Here's how the part is built. I have some questions about the finished solid (model axes, mm). A direction names the side the tool comes from. Round coordinates to 2 decimals unless told otherwise and drop trailing zeros. Loops run counter-clockwise (first coordinate to the right, second up) from the corner with the lowest first, then second, coordinate; pieces in that order, holes last. Notation, with made-up numbers: (-8.75, -9) - (0.25, -9) arc R16 ccw to (0.25, -3) - close; hole circle Ø5 at (89, 71.25). An arc over 180 degrees is marked (long way). Answer as a JSON object with one key per item and string values. Group by question number.
1) If we mould it in two halves opening along X, with no side actions, what happens to faces 4 (the face through (1.902, 0.986, -5.739)), 5 (the face through (0, 1, 16)), 6 (the face through (-4.766, 0.986, -1.475)), 7 (the face through (0, 8, 9))? For each: pulls with the +X half, pulls with the -X half, needs draft (parallel to the pull), parting line crosses it, or undercut.
2) I want a section at A-A, the plane z = 0. Please give me the cut outline in (x, y), then the cut area to 3 significant figures.
3) I want a section at C-C, the plane y = 1. Please give me the cut outline in (x, z), then the cut area to 3 significant figures.
4) If I drill on line 1 along X through (y, z) = (1.25, 0); line 2 along Z through (x, y) = (0, 0.5); line 3 along Y through (x, z) = (2, 14), over which ranges is the centre line in solid material (lowest first)? Write a range as [from, to].
5) Will these pins go through, and if not, where does the flat tip stop? P1, Ø4, axis at x = 0.5, z = 5.5, coming from the -Y side; P2, Ø2, axis at x = -5, y = 2, coming from the +Z side; P3, Ø1.6, axis at y = 1, z = 11.5, coming from the -X side; P4, Ø4, axis at x = -1, y = 7, coming from the -Z side.
6) Which directions (+Z, -Z, +X, -X, +Y, -Y) give clear straight access to the entire face, cutting with the end or side of a thin tool? Please do faces 1 (the face through (0.11, 7.415, 11.748)), 2 (the face through (-3, 1, 10)), 3 (the face through (3, 1, 10)).
7) I want a section at B-B, the plane x = -5. Please give me the cut outline in (y, z), then the cut area to 3 significant figures.
8) I want a section at D-D, the plane z = 9.25. Please give me the cut outline in (x, y), then the cut area to 3 significant figures.
from build123d import *

# Parameters (mm, degrees)
SKETCH_1_R      = 2
EXTRUDE_1_DEPTH = 2
SKETCH_2_R      = 2.5
EXTRUDE_2_DEPTH = 8


with BuildPart() as part:
    # 草图1 → 凸台-拉伸1 (new body)
    with BuildSketch(Plane(origin=(0, 0, 0), x_dir=(1, 0, 0), z_dir=(0, 1, 0))):
        with BuildLine():
            Line((3, -7.846018098), (3, -13))
            ThreePointArc((3, -13), (0, -16), (-3, -13))
            Line((-3, -13), (-3, -7.846018098))
            ThreePointArc((-3, -7.846018098), (-8.125792122, -2.128732579), (-6.461538462, 5.367356958))
            ThreePointArc((-6.461538462, 5.367356958), (-1.955292588, 5.784188007), (-1.538461538, 1.277942133))
            ThreePointArc((-1.538461538, 1.277942133), (0, -2), (1.538461538, 1.277942133))
            ThreePointArc((1.538461538, 1.277942133), (1.955292588, 5.784188007), (6.461538462, 5.367356958))
            ThreePointArc((6.461538462, 5.367356958), (8.125792122, -2.128732579), (3, -7.846018098))
        make_face()
        with Locations(Location((-4, 3.322649545, 0), (0, 0, 270))):
            Circle(SKETCH_1_R, mode=Mode.SUBTRACT)
        with Locations(Location((4, 3.322649545, 0), (0, 0, 270))):
            Circle(SKETCH_1_R, mode=Mode.SUBTRACT)
    extrude(amount=EXTRUDE_1_DEPTH)

    # 草图2 → 凸台-拉伸2 (add)
    with BuildSketch(Plane.XZ):
        with Locations(Location((0, 9.25, 0), (0, 0, 270))):
            Circle(SKETCH_2_R)
    extrude(amount=-EXTRUDE_2_DEPTH)

    # 草图7 → 旋转3 (revolve)
    with BuildSketch(Plane(origin=(0, 0, 11.498467043), x_dir=(0, 0, 1), z_dir=(-1, 0, 0)), mode=Mode.PRIVATE) as revolve_3_sk:
        Polygon((-2.248467043, 5.1), (0.251532957, 5.1), (0.351532957, 5.473205081), (0.351532957, 6.473205081), (0.251532957, 6.846410162), (-2.248467043, 6.846410162), align=None)
    revolve(revolve_3_sk.sketch.rotate(Axis((0, 2, 9.25), (0, 1, 0)), 180), axis=Axis((0, 2, 9.25), (0, 1, 0)))


solid = part.part
Outcome:
{
 "1": {"face 4": "undercut", "face 5": "parting line crosses it", "face 6": "undercut", "face 7": "needs draft"},
 "2": {"outline": "(-8.4, 0) - (-2, 0) - (-2, 2) - (-8.4, 2) - close; (2, 0) - (8.4, 0) - (8.4, 2) - (2, 2) - close", "area": "25.6 mm^2"},
 "3": {"outline": "(-6.46, -5.37) arc R3.2 ccw to (-1.54, -1.28) arc R2 cw (long way) to (1.54, -1.28) arc R3.2 ccw to (6.46, -5.37) arc R8.4 ccw to (3, 7.85) - (3, 13) arc R3 ccw to (-3, 13) - (-3, 7.85) arc R8.4 ccw to start; hole circle Ø4 at (-4, -3.32); hole circle Ø4 at (4, -3.32)", "area": "201 mm^2"},
 "4": {"line 1": "[-8.4, -2], [2, 8.4]", "line 2": "[2, 16]", "line 3": "[0, 2]"},
 "5": {"P1": "y = 0", "P2": "z = 7.39", "P3": "x = -3", "P4": "z = 6.65"},
 "6": {"face 1": "+Y", "face 2": "+Z, -X, +Y, -Y", "face 3": "+Z, +X, +Y, -Y"},
 "7": {"outline": "(0, -6.36) - (2, -6.36) - (2, -5.05) - (0, -5.05) - close; (0, -1.59) - (2, -1.59) - (2, 6.75) - (0, 6.75) - close", "area": "19.3 mm^2"},
 "8": {"outline": "(-3, 0) - (3, 0) - (3, 2) - (2.5, 2) - (2.5, 5.1) - (2.6, 5.47) - (2.6, 6.47) - (2.5, 6.85) - (2.5, 8) - (-2.5, 8) - (-2.5, 6.85) - (-2.6, 6.47) - (-2.6, 5.47) - (-2.5, 5.1) - (-2.5, 2) - (-3, 2) - close", "area": "42.3 mm^2"}
}
